Could you check a few things on this model? Use its own coordinates, in mm. Face numbers are marked on the shaded views. A direction names the side the tool comes from. Round coordinates to 2 decimals unless told otherwise and drop trailing zeros. Loops run counter-clockwise (first coordinate to the right, second up) from the corner with the lowest first, then second, coordinate; pieces in that order, holes last.
from build123d import *

# Parameters (mm, degrees)
SKETCH2_R               = 6
CUT_EXTRUDE1_DEPTH      = 33.5
CUT_EXTRUDE1_DEPTH_BACK = 33.5
SKETCH3_R               = 6
CUT_EXTRUDE2_DEPTH      = 30
SKETCH5_R               = 5.5
CUT_EXTRUDE4_DEPTH      = 5


with BuildPart() as part:
    # Sketch1 → Revolve2 (revolve)
    with BuildSketch(Plane.XY):
        Polygon((70.405866489, 0), (70.405866489, 18.292893219), (69.698759708, 19), (-86.594133511, 19), (-86.594133511, 22.5), (-96.594133511, 32.5), (-150.920978651, 32.5), (-156.594133511, 26.82684514), (-156.594133511, 11), (-169.594133511, 11), (-169.594133511, 0), align=None)
    revolve(axis=Axis((-169.594133511, 0, 0), (1, 0, 0)))

    # Sketch2 → Cut-Extrude1 (cut, two sides)
    with BuildSketch(Plane(origin=(0, 0, 0), x_dir=(1, 0, 0), z_dir=(0, 1, 0))) as cut_extrude1_sk:
        with Locations((-121.594133511, -1.00894074)):
            Circle(SKETCH2_R)
    extrude(amount=CUT_EXTRUDE1_DEPTH, mode=Mode.SUBTRACT)
    extrude(cut_extrude1_sk.sketch, amount=-CUT_EXTRUDE1_DEPTH_BACK, mode=Mode.SUBTRACT)

    # Sketch3 → Cut-Extrude2 (cut)
    with BuildSketch(Plane.ZY.offset(169.594133511)):
        Circle(SKETCH3_R)
    extrude(amount=-CUT_EXTRUDE2_DEPTH, mode=Mode.SUBTRACT)

    # Sketch5 → Cut-Extrude4 (cut)
    with BuildSketch(Plane.ZY.offset(139.594133511)):
        Circle(SKETCH5_R)
    extrude(amount=-CUT_EXTRUDE4_DEPTH, mode=Mode.SUBTRACT)


solid = part.part
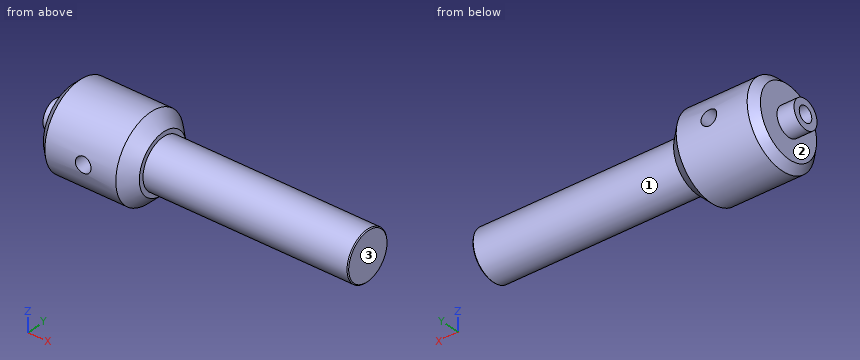
Item 1: If we section it at A-A, the plane x = -58.5: Please give me the cut outline in (y, z), then the cut area to 3 significant figures.
Results list:
outline: circle Ø38 at (0, 0)
area: 1,130 mm2
Item 2: For the marked faces 1, 2 and 3, which set-ups out of +Z, -Z, +X, -X, +Y, -Y let a thin tool reach every point of the face, with its end or its side?
Results list:
face 1: +X
face 2: -X
face 3: +Z, -Z, +X, +Y, -Y
Item 3: Will these pins go through, and if not, where does the flat tip stop? pin 1 (14 mm diameter, centred on x = -121.59, z = 1.01, fed in from -Y); pin 2 (4 mm diameter, centred on x = -130, z = -5, fed in from +Y); pin 3 (3.5 mm diameter, centred on y = 0.5, z = 1, fed in from -X); pin 4 (6 mm diameter, centred on y = -0.5, z = 2.5, fed in from -X).
Results list:
pin 1: stops at y = -32.5
pin 2: stops at y = 32.36
pin 3: stops at x = -134.59
pin 4: stops at x = -139.59
Item 4: If I drill on line 1 along Y through (x, z) = (-137.95, 0); line 2 along Y through (x, z) = (-145, 0); line 3 along X through (y, z) = (-13, 9.5), over which ranges is the centre line in solid material (lowest first)?
Results list:
line 1: y = -32.5 to -5.5, 5.5 to 32.5
line 2: y = -32.5 to -6, 6 to 32.5
line 3: x = -156.59 to 70.41
Item 5: If we section it at B-B, the plane x = -99.5: Please give me the cut outline in (y, z).
Results list:
outline: circle Ø65 at (0, 0)
